Build history of the part. All positions in model axes, mm. A direction names the side the tool comes from. Coordinates: 2 decimals unless noted, no trailing zeros. Order: outer loops, then holes, each group sorted by start corner. A loop starts at its lowest first (then second) coordinate and runs counter-clockwise, first axis right, second up. Notation, with made-up numbers: M -39.5,13.25 L 16.5,13.25 A23 ccw 16.5,27.25 Z; hole C -15,-21 d3. An arc over 180 degrees is marked long. Write item = value, one per line. Start each with the question number.
Q1. 3-axis set-ups, long thin cutter, end or side, ignore diameter. For faces 4 (the face through (-0.8, -1, 1)), 5 (the face through (2.89, -1.5, -0.07)): which of +Z, -Z, +X, -X, +Y, -Y reach the whole face in a straight line?
Q2. Drill centre lines: probe 1 along X at (y, z) = (-1, -1.25); probe 2 along Z at (x, y) = (5.25, 0); probe 3 along Y at (x, z) = (2.5, -1.25). Where is each one in solid material? Low to high.
Q3. Band-saw the part on A-A on y = 0. Write the cut outline in (x, z), plus the area to 3 significant figures.
Q4. Pin check, flat tips, straight feed: P1, Ø1.5, axis at y = -2.5, z = -2, coming from the +X side; P2, Ø3, axis at x = 2.5, z = 2.5, coming from the -Y side; P3, Ø1, axis at x = 2.5, z = -1.5, coming from the +Y side. Stop position of each tip, or through.
Q5. Band-saw the part on C-C on x = 1.5. Write the cut outline in (y, z), plus the area to 3 significant figures.
Q6. Pull direction Z, two halves, no side cores. Call faces 1 (the face through (6, 0, 0)), 2 (the face through (-0.197, 3.233, 1.341)), 3 (the face through (-0.4, 0, 0)): released by +Z, released by -Z, zero draft, split by the parting line, or undercut.
```python
from build123d import *

# Parameters (mm, degrees)
CUT_EXTRUDE1_DEPTH = 0.4


with BuildPart() as part:
    # Sketch1 → Revolve1 (revolve)
    with BuildSketch(Plane.XY):
        Polygon((-0.8, 0), (-0.8, 2.8), (-0.4, 3.5), (0, 3.5), (0, 1.5), (5.6935, 1.5), (6, 1.1935), (6, 0), align=None)
    revolve(axis=Axis((6, 0, 0), (-1, 0, 0)))

    # Sketch2 → Cut-Extrude1 (cut)
    with BuildSketch(Plane(origin=(-0.8, 0, 0), x_dir=(0, 0, -1), z_dir=(1, 0, 0))):
        with BuildLine():
            Line((-1.166666667, 0.233333357), (-1.166666667, -0.233333333))
            Line((-1.166666667, -0.233333333), (-0.46666669, -0.233333333))
            ThreePointArc((-0.46666669, -0.233333333), (-0.301675108, -0.301675084), (-0.233333357, -0.466666667))
            Line((-0.233333357, -0.466666667), (-0.233333357, -1.166666667))
            Line((-0.233333357, -1.166666667), (0.233333333, -1.166666667))
            Line((0.233333333, -1.166666667), (0.233333333, -0.466666667))
            ThreePointArc((0.233333333, -0.466666667), (0.301675084, -0.301675084), (0.466666667, -0.233333333))
            Line((0.466666667, -0.233333333), (1.166666667, -0.233333333))
            Line((1.166666667, -0.233333333), (1.166666667, 0.233333357))
            Line((1.166666667, 0.233333357), (0.466666667, 0.233333357))
            ThreePointArc((0.466666667, 0.233333357), (0.301675084, 0.301675108), (0.233333333, 0.46666669))
            Line((0.233333333, 0.46666669), (0.233333333, 1.166666667))
            Line((0.233333333, 1.166666667), (-0.233333357, 1.166666667))
            Line((-0.233333357, 1.166666667), (-0.233333357, 0.46666669))
            ThreePointArc((-0.233333357, 0.46666669), (-0.301675108, 0.301675108), (-0.46666669, 0.233333357))
            Line((-0.46666669, 0.233333357), (-1.166666667, 0.233333357))
        make_face()
    extrude(amount=CUT_EXTRUDE1_DEPTH, mode=Mode.SUBTRACT)


solid = part.part
```
Recorded:
q1.face_4 = +Z, -Z, -X, +Y, -Y
q1.face_5 = +X
q2.probe_1 = -0.8 to 0
q2.probe_2 = -1.5 to 1.5
q2.probe_3 = -0.83 to 0.83
q3.outline = M -0.8,-2.8 L -0.4,-3.5 L 0,-3.5 L 0,-1.5 L 5.69,-1.5 L 6,-1.19 L 6,1.19 L 5.69,1.5 L 0,1.5 L 0,3.5 L -0.4,3.5 L -0.8,2.8 L -0.8,1.17 L -0.4,1.17 L -0.4,-1.17 L -0.8,-1.17 Z
q3.area = 22.3 mm2
q4.P1 = 0
q4.P2 = -1.12
q4.P3 = 1.12
q5.outline = C 0,0 d3
q5.area = 7.07 mm2
q6.face_1 = zero draft
q6.face_2 = split by the parting line
q6.face_3 = undercut
